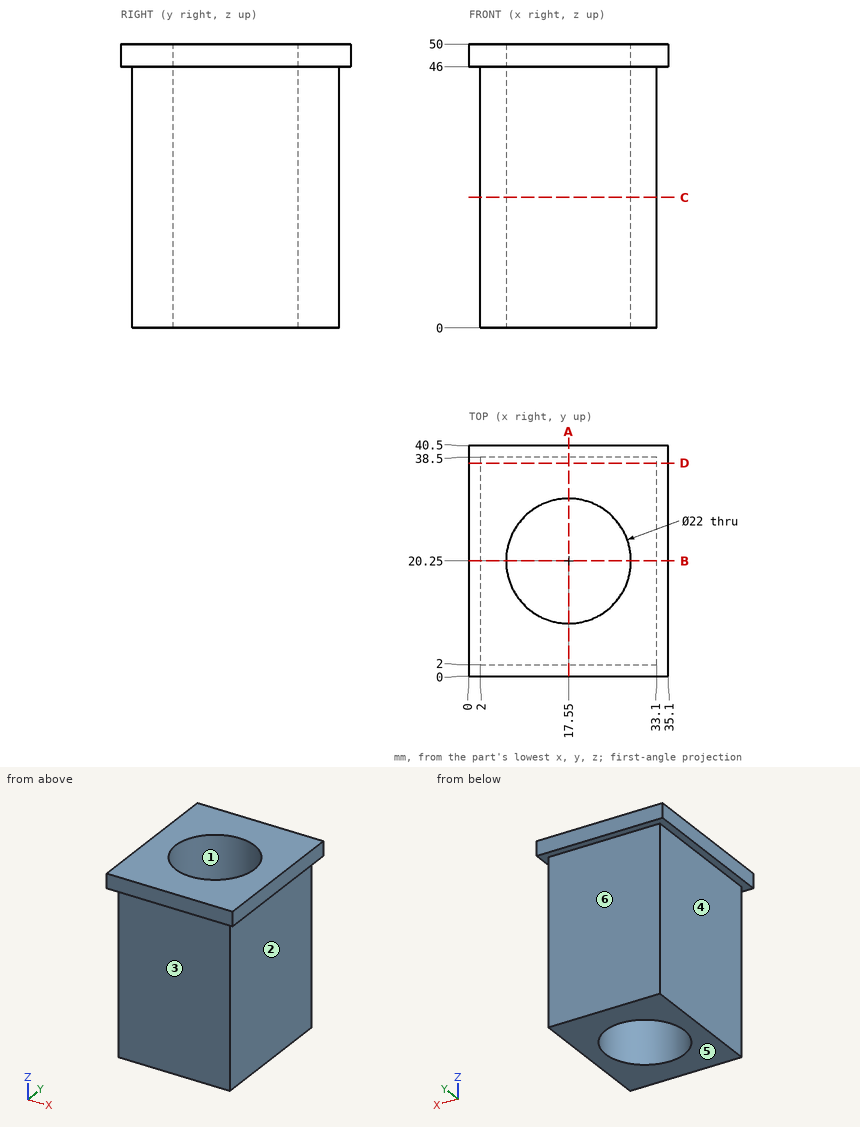
Print and shaded views of the part. All mm, measured from the part's lowest x, y and z. A direction names the side the tool comes from. Round coordinates to 2 decimals unless told otherwise and drop trailing zeros. Write each loop counter-clockwise with the first axis right and the second up, starting at its lowest first coordinate (ties: lowest second). Pieces come first, ordered by that corner, then holes. Notation, with made-up numbers: (81.5, -37) -> (91.5, -37) arc R21 cw to (91.5, 0) -> close; hole circle Ø11 at (-21.75, 37). An arc over 180 degrees is marked (long way). Return JSON: item names as keys, results as strings. Group by question number.
Q1. Saw through at D-D on y = 37.5. Write the cut outline in (x, z).
Q2. Which spindle directions (+Z, -Z, +X, -X, +Y, -Y) get a long thin tool onto all of the face, cutting with end or side? Do the marked faces 5 and 6. Say none if no direction does.
Q3. Mould opens along X. For the marked faces 1, 2, 3 and 4 say: pulls with the +X half, pulls with the -X half, needs draft (parallel to the pull), parting line crosses it, or undercut.
Q4. Saw through at B-B on y = 20.25. Write the cut outline in (x, z), plus the area to 3 significant figures.
Q5. Saw through at A-A on x = 17.55. Write the cut outline in (y, z), plus the area to 3 significant figures.
Q6. Saw through at C-C on z = 23. Write the cut outline in (x, y).
Q7. Probe L1, parallel to Y at x = 18, z = 47; L2, parallel to Y at x = 17.55, z = 35.5; L3, parallel to X at y = 20, z = 10. List the from-to ranges inside material, lowest first. Write a range as [from, to].
Q8. Pin check, flat tips, straight feed: pin 1 (4 mm diameter, centred on x = 9.5, z = 14.5, fed in from +Y); pin 2 (8 mm diameter, centred on y = 8, z = 35, fed in from +X); pin 3 (8 mm diameter, centred on y = 35, z = 39, fed in from -X). Stop position of each tip, or through.
Answer:
{
 "1": {"outline": "(0, 46) -> (2, 46) -> (2, 0) -> (33.1, 0) -> (33.1, 46) -> (35.1, 46) -> (35.1, 50) -> (0, 50) -> close"},
 "2": {"face 5": "-Z, +X, -X, +Y, -Y", "face 6": "-Z, +X, -X, +Y"},
 "3": {"face 1": "undercut", "face 2": "pulls with the +X half", "face 3": "needs draft", "face 4": "pulls with the -X half"},
 "4": {"outline": "(0, 46) -> (2, 46) -> (2, 0) -> (6.55, 0) -> (6.55, 50) -> (0, 50) -> close; (28.55, 0) -> (33.1, 0) -> (33.1, 46) -> (35.1, 46) -> (35.1, 50) -> (28.55, 50) -> close", "area": "471 mm2"},
 "5": {"outline": "(0, 46) -> (2, 46) -> (2, 0) -> (9.25, 0) -> (9.25, 50) -> (0, 50) -> close; (31.25, 0) -> (38.5, 0) -> (38.5, 46) -> (40.5, 46) -> (40.5, 50) -> (31.25, 50) -> close", "area": "741 mm2"},
 "6": {"outline": "(2, 2) -> (33.1, 2) -> (33.1, 38.5) -> (2, 38.5) -> close; hole circle Ø22 at (17.55, 20.25)"},
 "7": {"L1": "[0, 9.26], [31.24, 40.5]", "L2": "[2, 9.25], [31.25, 38.5]", "L3": "[2, 6.55], [28.55, 33.1]"},
 "8": {"pin 1": "y = 38.5", "pin 2": "x = 33.1", "pin 3": "x = 2"}
}
